Work out the finished part from the listing and answer in its coordinate system (mm). Face numbers are marked on the shaded views. A direction names the side the tool comes from. Round coordinates to 2 decimals unless told otherwise and drop trailing zeros. Write each loop counter-clockwise with the first axis right and the second up, starting at its lowest first coordinate (ties: lowest second). Pieces come first, ordered by that corner, then holes.
1. Determine the mould class of the marked faces 4 and 5 for opening direction Z: pulls with the +Z half, pulls with the -Z half, needs draft (parallel to the pull), parting line crosses it, or undercut.
2. Find section A-A (x = -9.15). Write down the section's boundary in (y, z), and give its area (3 significant figures).
3. Straight lines are drawn through the part: probe 1 along Z at (x, y) = (-10.4, 0); probe 2 along Y at (x, z) = (-9.5, -10). For each, find the intervals that lie inside material, in ascending order.
4. A tool of negligible diameter and unlimited length cuts with its end or side. For the marked faces 1, 2 and 3, from which of +Z, -Z, +X, -X, +Y, -Y can it reach the whole face along a straight path? Write none if from no direction.
5. Find section B-B (y = 0). Write down the section's boundary in (x, z) (3 decimals).
6. Find section D-D (y = -8.5). Write down the section's boundary in (x, z) (3 decimals).
7. A flat-ended cylindrical pin translates along its axis: pin 1 Ø3.5 at (y, z) = (-4.5, 1.5) entering from +X. Find the tip coordinate at first contact, or state that the pin passes through.
8. Find section C-C (z = -9). Write down the section's boundary in (x, y) (3 decimals), and give its area (3 significant figures).
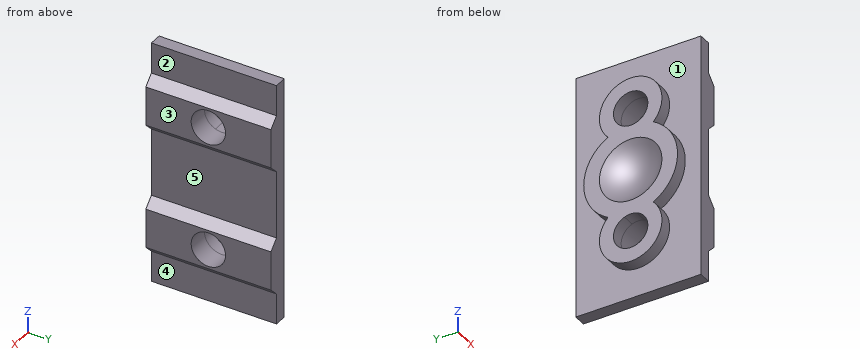
```python
from build123d import *

# Parameters (mm, degrees)
F2_DEPTH  = 10
F3_R      = 7.5
F4_DEPTH  = 2
F8_D      = 5.5
F8_DEPTH  = 3.456
F9_R      = 2.75
F10_DEPTH = 25
F11_R     = 5
F11_R_2   = 2.75
F12_DEPTH = 2


with BuildPart() as f2:
    # F1 (on Front) → F2 (new body, symmetric)
    with BuildSketch(Plane.XZ):
        Polygon((-10, -5.42), (-10, 5.42), (-8.545, 6.875), (-8.545, 13.125), (-10, 14.58), (-10, 19.5), (-12, 19.5), (-12, -19.5), (-10, -19.5), (-10, -14.58), (-8.545, -13.125), (-8.545, -6.875), align=None)
    extrude(amount=F2_DEPTH, both=True)

    # F3 (on face) → F4 (join)
    with BuildSketch(Plane(origin=(-12, 0, 0), x_dir=(0, -1, 0), z_dir=(-1, 0, 0))):
        Circle(F3_R)
    extrude(amount=F4_DEPTH)

    # F5 (on Top) → F6 (revolve, cut)
    with BuildSketch(Plane.XY):
        with BuildLine():
            Line((-14, 0), (-14, -5))
            ThreePointArc((-14, -5), (-12.5185439911, -2.6925824036), (-12, 0))
            Line((-12, 0), (-14, 0))
        make_face()
    revolve(axis=Axis((-13, 0, 0), (-1, 0, 0)), mode=Mode.SUBTRACT)

    # F8 (through all, one way)
    with BuildSketch(Plane(origin=(-12, 0, 0), x_dir=(0, -1, 0), z_dir=(-1, 0, 0))):
        with Locations((0, 10), (0, -10)):
            Circle(F8_D / 2)
    extrude(amount=-F8_DEPTH, mode=Mode.SUBTRACT)

    # F9 (on face) → F10 (cut)
    with BuildSketch(Plane.YZ.offset(-8.545)):
        with Locations((0, 10)):
            Circle(F9_R)
        with Locations((0, -10)):
            Circle(F9_R)
    extrude(amount=-F10_DEPTH, mode=Mode.SUBTRACT)

    # F11 (on face) → F12 (join, through all)
    with BuildSketch(Plane(origin=(-12, 0, 0), x_dir=(0, -1, 0), z_dir=(-1, 0, 0))):
        with Locations((0, 10)):
            Circle(F11_R)
        with Locations((0, 10)):
            Circle(F11_R_2, mode=Mode.SUBTRACT)
        with Locations((0, -10)):
            Circle(F11_R)
        with Locations((0, -10)):
            Circle(F11_R_2, mode=Mode.SUBTRACT)
    extrude(amount=F12_DEPTH)


solid = f2.part
```
Worked answers:
1. face 4: needs draft
1. face 5: undercut
2. outline: (-10, -13.73) - (10, -13.73) - (10, -6.27) - (-10, -6.27) - close; (-10, 6.27) - (10, 6.27) - (10, 13.73) - (-10, 13.73) - close; hole circle Ø5.5 at (0, -10); hole circle Ø5.5 at (0, 10)
2. area: 251 mm2
3. probe 1: z = -19.5 to -12.75, -7.25 to 7.25, 12.75 to 19.5
3. probe 2: y = -10 to -2.75, 2.75 to 10
4. face 1: -X
4. face 2: +Z, +X, +Y, -Y
4. face 3: +Z, -Z, +X, +Y, -Y
5. outline: (-14, -15) - (-12, -15) - (-12, -19.5) - (-10, -19.5) - (-10, -14.58) - (-8.545, -13.125) - (-8.545, -12.75) - (-14, -12.75) - close; (-14, -7.25) - (-8.545, -7.25) - (-8.545, -6.875) - (-10, -5.42) - (-10, 5.42) - (-8.545, 6.875) - (-8.545, 7.25) - (-14, 7.25) - (-14, 5) arc R7.25 cw to (-14, -5) - close; (-14, 12.75) - (-8.545, 12.75) - (-8.545, 13.125) - (-10, 14.58) - (-10, 19.5) - (-12, 19.5) - (-12, 15) - (-14, 15) - close
6. outline: (-12, -19.5) - (-10, -19.5) - (-10, -14.58) - (-8.545, -13.125) - (-8.545, -6.875) - (-10, -5.42) - (-10, 5.42) - (-8.545, 6.875) - (-8.545, 13.125) - (-10, 14.58) - (-10, 19.5) - (-12, 19.5) - close
7. pin 1: stops at x = -10
8. outline: (-14, -4.899) - (-12, -4.899) - (-12, -10) - (-8.545, -10) - (-8.545, -2.562) - (-14, -2.562) - close; (-14, 2.562) - (-8.545, 2.562) - (-8.545, 10) - (-12, 10) - (-12, 4.899) - (-14, 4.899) - close
8. area: 60.7 mm2
